Verification items for the finished model (mm, model axes). Face numbers are marked on the shaded views. Give positions to 0.01 mm unless a question says otherwise; leave off trailing zeros. Write each loop counter-clockwise with the first axis right and the second up, starting at its lowest first coordinate (ties: lowest second). Pieces come first, ordered by that corner, then holes. Notation, with made-up numbers: (-38.5, -11.5) -> (-13.5, -11.5) arc R26 cw to (-13.5, 19.5) -> close; hole circle Ø3 at (-12, 49). An arc over 180 degrees is marked (long way). Use CSV: the item, a comma, the result in double quotes. Start each with the question number.
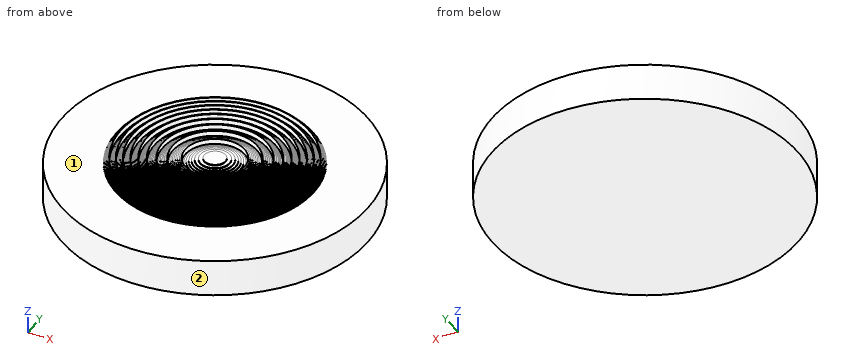
```python
from build123d import *


with BuildPart() as f1:
    # F0 (on Front) → F1 (revolve)
    with BuildSketch(Plane.XZ):
        Polygon((0, 3.507), (0, 0), (12.7, 0), (12.7, 3.063), (8.291, 3.063), (8.232, 3.063), (8.232, 3.127), (8.173, 3.127), (8.173, 3.19), (8.114, 3.19), (8.114, 3.253), (8.055, 3.253), (8.055, 3.317), (7.995, 3.317), (7.995, 3.38), (7.935, 3.38), (7.935, 3.443), (7.875, 3.443), (7.875, 3.507), (7.814, 3.507), (7.814, 3.063), (7.753, 3.063), (7.753, 3.127), (7.692, 3.127), (7.692, 3.19), (7.631, 3.19), (7.631, 3.253), (7.569, 3.253), (7.569, 3.317), (7.507, 3.317), (7.507, 3.38), (7.444, 3.38), (7.444, 3.443), (7.382, 3.443), (7.382, 3.507), (7.319, 3.507), (7.319, 3.063), (7.255, 3.063), (7.255, 3.127), (7.191, 3.127), (7.191, 3.19), (7.127, 3.19), (7.127, 3.253), (7.062, 3.253), (7.062, 3.317), (6.998, 3.317), (6.998, 3.38), (6.932, 3.38), (6.932, 3.443), (6.866, 3.443), (6.866, 3.507), (6.8, 3.507), (6.8, 3.053), (6.733, 3.053), (6.733, 3.127), (6.666, 3.127), (6.666, 3.19), (6.599, 3.19), (6.599, 3.253), (6.53, 3.253), (6.53, 3.317), (6.462, 3.317), (6.462, 3.38), (6.393, 3.38), (6.393, 3.443), (6.323, 3.443), (6.323, 3.507), (6.253, 3.507), (6.253, 3.063), (6.182, 3.063), (6.182, 3.127), (6.111, 3.127), (6.111, 3.19), (6.039, 3.19), (6.039, 3.253), (5.966, 3.253), (5.966, 3.317), (5.893, 3.317), (5.893, 3.38), (5.819, 3.38), (5.819, 3.443), (5.744, 3.443), (5.744, 3.507), (5.669, 3.507), (5.669, 3.063), (5.593, 3.063), (5.593, 3.127), (5.516, 3.127), (5.516, 3.19), (5.438, 3.19), (5.438, 3.253), (5.359, 3.253), (5.359, 3.317), (5.28, 3.317), (5.28, 3.38), (5.199, 3.38), (5.199, 3.443), (5.117, 3.443), (5.117, 3.507), (5.035, 3.507), (5.035, 3.063), (4.951, 3.063), (4.951, 3.127), (4.866, 3.127), (4.866, 3.19), (4.78, 3.19), (4.78, 3.253), (4.693, 3.253), (4.693, 3.317), (4.604, 3.317), (4.604, 3.38), (4.514, 3.38), (4.514, 3.443), (4.423, 3.443), (4.423, 3.507), (4.33, 3.507), (4.33, 3.063), (4.235, 3.063), (4.235, 3.127), (4.138, 3.127), (4.138, 3.19), (4.039, 3.19), (4.039, 3.253), (3.938, 3.253), (3.938, 3.317), (3.835, 3.317), (3.835, 3.38), (3.729, 3.38), (3.729, 3.443), (3.621, 3.443), (3.621, 3.507), (3.51, 3.507), (3.51, 3.063), (3.395, 3.063), (3.395, 3.127), (3.277, 3.127), (3.277, 3.19), (3.155, 3.19), (3.155, 3.253), (3.028, 3.253), (3.028, 3.317), (2.897, 3.317), (2.897, 3.38), (2.759, 3.38), (2.759, 3.443), (2.615, 3.443), (2.615, 3.507), (2.464, 3.507), (2.464, 3.063), (2.302, 3.063), (2.302, 3.127), (2.13, 3.127), (2.13, 3.19), (1.942, 3.19), (1.942, 3.253), (1.735, 3.253), (1.735, 3.317), (1.502, 3.317), (1.502, 3.38), (1.225, 3.38), (1.225, 3.443), (0.8865, 3.443), (0.8865, 3.507), align=None)
    revolve(axis=Axis((0, 0, 1.7535), (0, 0, 1)))


solid = f1.part
```
(1) Section check A-A on z = 1.85. Record the cut outline in (x, y).
(2) Draft check along X on the marked faces 1 and 2. Enter one of: released by +X, released by -X, zero draft, split by the parting line, or undercut.
(3) Go/stop test with flat-tipped pins: pin 1 (2 mm diameter, centred on x = -7, z = 0.5, fed in from -Y); pin 2 (2 mm diameter, centred on x = -8.5, z = 3, fed in from -Y); pin 3 (8 mm diameter, centred on x = -8.5, y = -9.5, fed in from +Z). Record where each tip stops, or that it passes through.
(4) Section check B-B on y = 11.25. Record the cut outline in (x, z).
(5) Thickness scan on line 1 (Z direction, x = 6, y = 8.25); line 2 (Y direction, x = 7.5, z = 1.2); line 3 (Y direction, x = 10.5, z = 1.05). Record the ranges inside material, lowest first. Write a range as from..to.
Data:
1,outline,"circle Ø25.4 at (0, 0)"
2,face 1,"zero draft"
2,face 2,"split by the parting line"
3,pin 1,"stops at y = -11.19"
3,pin 2,"stops at y = -10.25"
3,pin 3,"stops at z = 3.06"
4,outline,"(-5.89, 0) -> (5.89, 0) -> (5.89, 3.06) -> (-5.89, 3.06) -> close"
5,line 1,"z = 0..3.06"
5,line 2,"y = -10.25..10.25"
5,line 3,"y = -7.14..7.14"
